from build123d import *

# Parameters (mm, degrees)
BOSS_EXTRUDE1_DEPTH = 5
SKETCH2_R           = 1.435
BOSS_EXTRUDE2_DEPTH = 3.5
BOSS_EXTRUDE3_START = 3.5
SKETCH3_R           = 1.435
BOSS_EXTRUDE3_DEPTH = 3.5


with BuildPart() as part:
    # Sketch1 → Boss-Extrude1 (new body)
    with BuildSketch(Plane.XY):
        Polygon((-45, 17.5), (-45, -17.5), (-38, -17.5), (-38, -3.5), (-24, -3.5), (-24, -17.5), (-5, -17.5), (5, -17.5), (45, -17.5), (45, 17.5), align=None)
    extrude(amount=BOSS_EXTRUDE1_DEPTH)

    # Sketch2 → Boss-Extrude2 (add)
    with BuildSketch(Plane(origin=(45, 0, 0), x_dir=(0, 0, -1), z_dir=(1, 0, 0))):
        with Locations(Location((-2.5, 9.5, 0), (0, 0, 180))):
            Circle(SKETCH2_R)
        with Locations(Location((-2.5, -9.5, 0), (0, 0, 180))):
            Circle(SKETCH2_R)
    extrude(amount=BOSS_EXTRUDE2_DEPTH)

    # Sketch3 → Boss-Extrude3 (add)
    with BuildSketch(Plane.ZY.offset(45).offset(BOSS_EXTRUDE3_START)):
        with Locations((2.5, 9.5)):
            Circle(SKETCH3_R)
        with Locations((2.5, -9.5)):
            Circle(SKETCH3_R)
    extrude(amount=-BOSS_EXTRUDE3_DEPTH)


solid = part.part
Source: CAD feature listing. Evaluate the final solid. Frame: model axes, mm. A direction names the side the tool comes from. Coordinates: 2 decimals unless noted, no trailing zeros. Order: outer loops, then holes, each group sorted by start corner. A loop starts at its lowest first (then second) coordinate and runs counter-clockwise, first axis right, second up. Notation, with made-up numbers: M 0,51 L 22,51 A32 ccw 22,90 Z; hole C 1.5,25 d1. An arc over 180 degrees is marked long. Write each question's results on one line, items separated by ' | '. Start each with the question number.
1. Section D-D, the plane y = 9.5. Return the cut outline in (x, z) (3 decimals).
2. Section C-C, the plane y = -9.5. Return the cut outline in (x, z) (3 decimals), then the cut area to 3 significant figures.
3. Section B-B, the plane z = 2.5. Return the cut outline in (x, y) (3 decimals).
4. Section A-A, the plane y = -14. Return the cut outline in (x, z), then the cut area to 3 significant figures.
5. Draft query along Y for faces 6 (the face through (1, 17.5, 2)), 7 (the face through (46.73, 10.9, 2.19)), 8 (the face through (-38, -11, 2)). Return one class per face: +Y half, -Y half, draft (parallel to the pull), parting line (faces both ways), or undercut.
6. Reachability of faces 1 (the face through (46.73, -8.1, 2.19)), 2 (the face through (-46.77, 8.1, 2.19)), 3 (the face through (-1, 0, 5)), 4 (the face through (48.5, 9, 2)), 5 (the face through (-31, -3.5, 2)) from +Z, -Z, +X, -X, +Y, -Y: full face, straight path, thin tool, end or side. Return the list, or none.
7. Material intervals for L1, parallel to X at y = -8, z = 2.25; L2, parallel to X at y = 6, z = 1.8; L3, parallel to X at y = -10.5, z = 2.45, sorted ascending.
8. Pin query (flat end, axial travel): pin 1 (2.5 mm diameter, centred on y = -2, z = 2, fed in from +X). Return the tip coordinate at first contact, or that it passes through.
Solution:
1) outline: M -48.5,1.065 L -45,1.065 L -45,0 L 45,0 L 45,1.065 L 48.5,1.065 L 48.5,3.935 L 45,3.935 L 45,5 L -45,5 L -45,3.935 L -48.5,3.935 Z
2) outline: M -48.5,1.065 L -45,1.065 L -45,0 L -38,0 L -38,5 L -45,5 L -45,3.935 L -48.5,3.935 Z; M -24,0 L 45,0 L 45,1.065 L 48.5,1.065 L 48.5,3.935 L 45,3.935 L 45,5 L -24,5 Z | area: 400 mm²
3) outline: M -48.5,-10.935 L -45,-10.935 L -45,-17.5 L -38,-17.5 L -38,-3.5 L -24,-3.5 L -24,-17.5 L 45,-17.5 L 45,-10.935 L 48.5,-10.935 L 48.5,-8.065 L 45,-8.065 L 45,8.065 L 48.5,8.065 L 48.5,10.935 L 45,10.935 L 45,17.5 L -45,17.5 L -45,10.935 L -48.5,10.935 L -48.5,8.065 L -45,8.065 L -45,-8.065 L -48.5,-8.065 Z
4) outline: M -45,0 L -38,0 L -38,5 L -45,5 Z; M -24,0 L 45,0 L 45,5 L -24,5 Z | area: 380 mm²
5) face 6: +Y half | face 7: undercut | face 8: draft
6) face 1: +X | face 2: -X | face 3: +Z, +X, -X, +Y, -Y | face 4: +Z, -Z, +X, +Y, -Y | face 5: +Z, -Z, -Y
7) L1: -45 to -38, -24 to 45 | L2: -45 to 45 | L3: -48.5 to -38, -24 to 48.5
8) pin 1: x = 45
